Work out the finished part from the listing and answer in its coordinate system (mm). A direction names the side the tool comes from. Round coordinates to 2 decimals unless told otherwise and drop trailing zeros. Write each loop counter-clockwise with the first axis right and the second up, starting at its lowest first coordinate (ties: lowest second). Pieces come first, ordered by that corner, then holes.
from build123d import *

# Parameters (mm, degrees)
F1_DEPTH = 15.24
F2_W     = 19.2376272753
F2_H     = 15.0951566175
F3_DEPTH = 5.08
F4_SIZE2 = 4.3994090512
F4_SIZE  = 7.62
F5_W     = 20.32
F5_H     = 41.094693502
F6_DEPTH = 7.62


with BuildPart() as f1:
    # F0 (on Top) → F1 (new body)
    with BuildSketch(Plane.XY):
        Polygon((-13.5031091049, 27.9268901795), (-10.1887094788, 14.7920455784), (-7.6487094788, 14.7920455784), (-7.6487094788, 19.1914546296), align=None)
        Polygon((-7.6487094788, 14.7920455784), (-10.1887094788, 14.7920455784), (-10.1887094788, -38.9519235189), (10.1312905212, -38.9519235189), (10.1312905212, 14.7920455784), (7.5912905212, 14.7920455784), (7.5912905212, 10.3926365271), (-0.0287094788, 5.9932274759), (-7.6487094788, 10.3926365271), align=None)
        Polygon((7.5912905212, 14.7920455784), (10.1312905212, 14.7920455784), (13.5031156242, 27.9268901795), (7.5912905212, 19.1914546296), align=None)
    extrude(amount=F1_DEPTH)

    # F2 (on face) → F3 (join)
    with BuildSketch(Plane.XY.offset(15.24)):
        with Locations((-0.1635341905, 12.2919357382)):
            Rectangle(F2_W, F2_H)
    extrude(amount=-F3_DEPTH)

    # F4
    f4_edges = [f1.edges().sort_by_distance(p)[0] for p in [
        (-0.026579, 19.839514, 10.16),
    ]]
    f4_side = f1.faces().sort_by_distance((-0.028648, 13.956011, 10.16))[0]
    chamfer(f4_edges, length=F4_SIZE, length2=F4_SIZE2, reference=f4_side)

    # F5 (on face) → F6 (cut)
    with BuildSketch(Plane(origin=(0, 0, 0), x_dir=(1, 0, 0), z_dir=(0, 0, -1))):
        with Locations((-0.0287094788, 18.4045767679)):
            Rectangle(F5_W, F5_H)
    extrude(amount=-F6_DEPTH, mode=Mode.SUBTRACT)


solid = f1.part
Q1. The mould has two halves that part along X. Classify faces 4 (the face through (10.131, -6, 11)), 5 (the face through (-3.785, 8.162, 5.009)), 6 (the face through (-10.189, -6, 11)): +X half, -X half, draft (parallel to the pull), parting line (faces both ways), or undercut.
Q2. A tool of negligible diameter and unlimited length cuts with its end or side. For faces 1 (the face through (-0.1, 16.1, 12.4)), 2 (the face through (0, 2.143, 4)), 3 (the face through (-3, 7, 0)), from which of +Z, -Z, +X, -X, +Y, -Y can it reach the whole face along a straight path? Write none if from no direction.
Q3. Given pin 1 (8 mm diameter, centred on y = 6.5, z = 10.5, fed in from +X); pin 2 (7.5 mm diameter, centred on y = -1, z = 11, fed in from -X); pin 3 (5 mm diameter, centred on x = 0.5, y = -2, fed in from -Z), each flat-ended and moving along its own axis, determine where each tip first touches the part or whether it passes through.
Q4. Find section C-C (x = -3). Determine the outline of the cut face in (y, z), plus the area to 3 significant figures.
Q5. Find section D-D (y = 14). Determine the outline of the cut face in (x, z), plus the area to 3 significant figures.
Q6. Find section A-A (y = 24.5). Determine the outline of the cut face in (x, z).
Q7. Find section B-B (z = 9.25). Determine the outline of the cut face in (x, y), plus the area to 3 significant figures.
Q8. Find the intervals of material crossed by L1, parallel to Z at x = 0, y = 12; L2, parallel to X at y = -14.5, z = 11.25; L3, parallel to Z at x = -5, y = -20.5, in increasing order.
Report:
1. face 4: +X half
1. face 5: undercut
1. face 6: -X half
2. face 1: -Z, +Y
2. face 2: -Z, +X, -X, -Y
2. face 3: -Z, +X, -X, +Y, -Y
3. pin 1: stops at x = 10.13
3. pin 2: stops at x = -10.19
3. pin 3: stops at z = 7.62
4. outline: (-38.95, 7.62) - (2.14, 7.62) - (2.14, 0) - (7.71, 0) - (7.71, 10.16) - (12.22, 10.16) - (19.84, 14.56) - (19.84, 15.24) - (-38.95, 15.24) - close
4. area: 443 mm2
5. outline: (-10.19, 0) - (-7.65, 0) - (-7.65, 11.19) - (7.59, 11.19) - (7.59, 0) - (10.13, 0) - (10.13, 15.24) - (-10.19, 15.24) - close
5. area: 139 mm2
6. outline: (-12.64, 0) - (-11.21, 0) - (-11.21, 15.24) - (-12.64, 15.24) - close; (11.18, 0) - (12.62, 0) - (12.62, 15.24) - (11.18, 15.24) - close
7. outline: (-13.5, 27.93) - (-10.19, 14.79) - (-10.19, -38.95) - (10.13, -38.95) - (10.13, 14.79) - (13.5, 27.93) - (7.59, 19.19) - (7.59, 10.39) - (-0.03, 5.99) - (-7.65, 10.39) - (-7.65, 19.19) - close
7. area: 1,050 mm2
8. L1: z = 10.16 to 15.24
8. L2: x = -10.19 to 10.13
8. L3: z = 7.62 to 15.24
